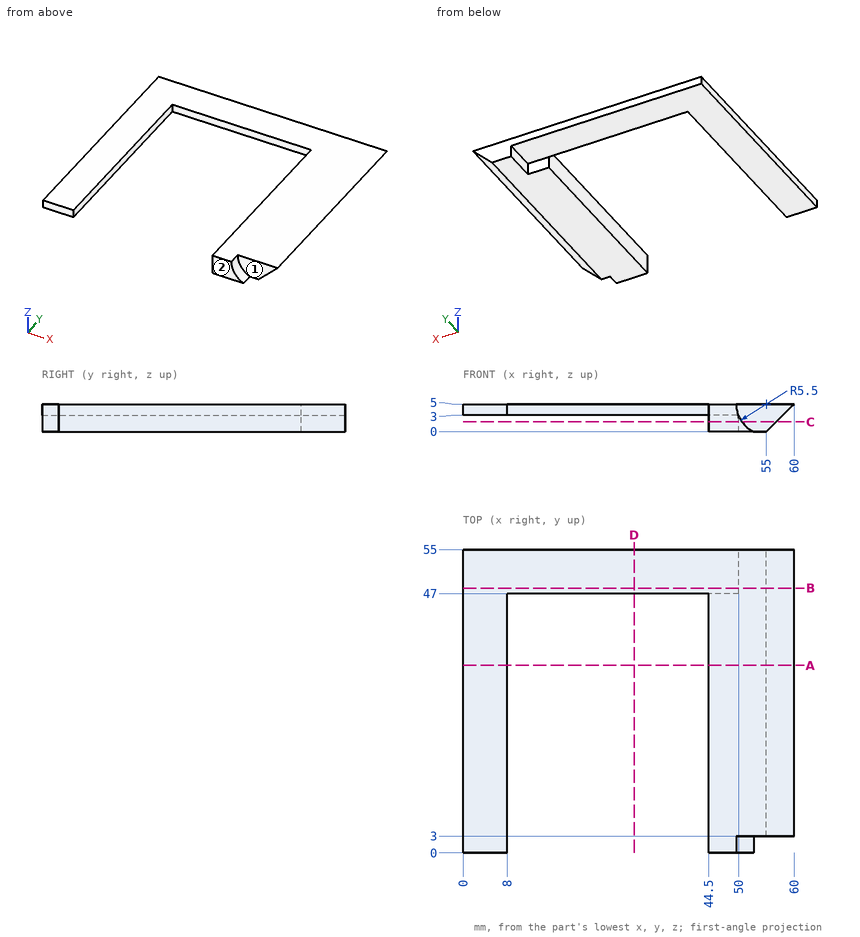
Input: dimensioned drawing with shaded views. Units: mm. Origin: part minimum x, y, z. A direction names the side the tool comes from. Round coordinates to 2 decimals unless told otherwise and drop trailing zeros. Write each loop counter-clockwise with the first axis right and the second up, starting at its lowest first coordinate (ties: lowest second). Pieces come first, ordered by that corner, then holes. Notation, with made-up numbers: (-18.75, 9.5) - (6.25, 9.5) arc R11 ccw to (6.25, 26.5) - close; hole circle Ø10 at (63.5, 29.25). An arc over 180 degrees is marked (long way). Write item = value, one per line.
(1) Access query for the marked faces 1 and 2. Directions: +Z, -Z, +X, -X, +Y, -Y. A direction counts if a zero-diameter tool reaches every point of the face in a straight line with its end or side. Return the directions, or none.
Geometry check:
face_1 = +Z, +X, -Y
face_2 = +Z, -Z, +X, -X, -Y
(2) Section query B-B on y = 48. Output: boundary loops of the cut face in (x, z), then the cut area to 4 significant figures.
Geometry check:
outline = (0, 3) - (50, 3) - (50, 0) - (55, 0) - (60, 5) - (0, 5) - close
area = 137.5 mm^2
(3) Section query C-C on z = 1.75. Output: boundary loops of the cut face in (x, y).
Geometry check:
outline = (44.5, 0) - (50.56, 0) - (50.56, 3) - (56.75, 3) - (56.75, 55) - (50, 55) - (50, 47) - (44.5, 47) - close
(4) Contact query for flat-ended pins moving along their axis: pin 1 Ø1 at (x, z) = (21, 3.5) entering from -Y; pin 2 Ø1.5 at (y, z) = (40, 3.5) entering from +X; pin 3 Ø3 at (y, z) = (37, 3) entering from +X. Output: stop coordinate, or through.
Geometry check:
pin_1 = 47
pin_2 = 59.25
pin_3 = 59.5
(5) Material intervals for probe 1 along Y at (x, z) = (55.5, 1.4); probe 2 along Z at (x, y) = (6.5, 30); probe 3 along X at (y, z) = (24, 4), sorted ascending.
Geometry check:
probe_1 = 3 to 55
probe_2 = 3 to 5
probe_3 = 0 to 8, 44.5 to 59
(6) Section query D-D on x = 31. Output: boundary loops of the cut face in (y, z).
Geometry check:
outline = (47, 3) - (55, 3) - (55, 5) - (47, 5) - close
(7) Section query A-A on y = 34. Output: boundary loops of the cut face in (x, z).
Geometry check:
outline = (0, 3) - (8, 3) - (8, 5) - (0, 5) - close; (44.5, 0) - (55, 0) - (60, 5) - (44.5, 5) - close
